Can you work these out from the drawing? Everything is in mm from the part's minimum corner. A direction names the side the tool comes from. Coordinates: 2 decimals unless noted, no trailing zeros. Write each loop counter-clockwise with the first axis right and the second up, starting at its lowest first coordinate (ties: lowest second). Pieces come first, ordered by that corner, then holes. Notation, with made-up numbers: (88, 85.25) -> (108, 85.25) arc R9 ccw to (108, 90.25) -> close; hole circle Ø3 at (-9.5, 88). An arc over 180 degrees is marked (long way). Use CSV: the item, a comma, the result in double quotes. Start each with the question number.
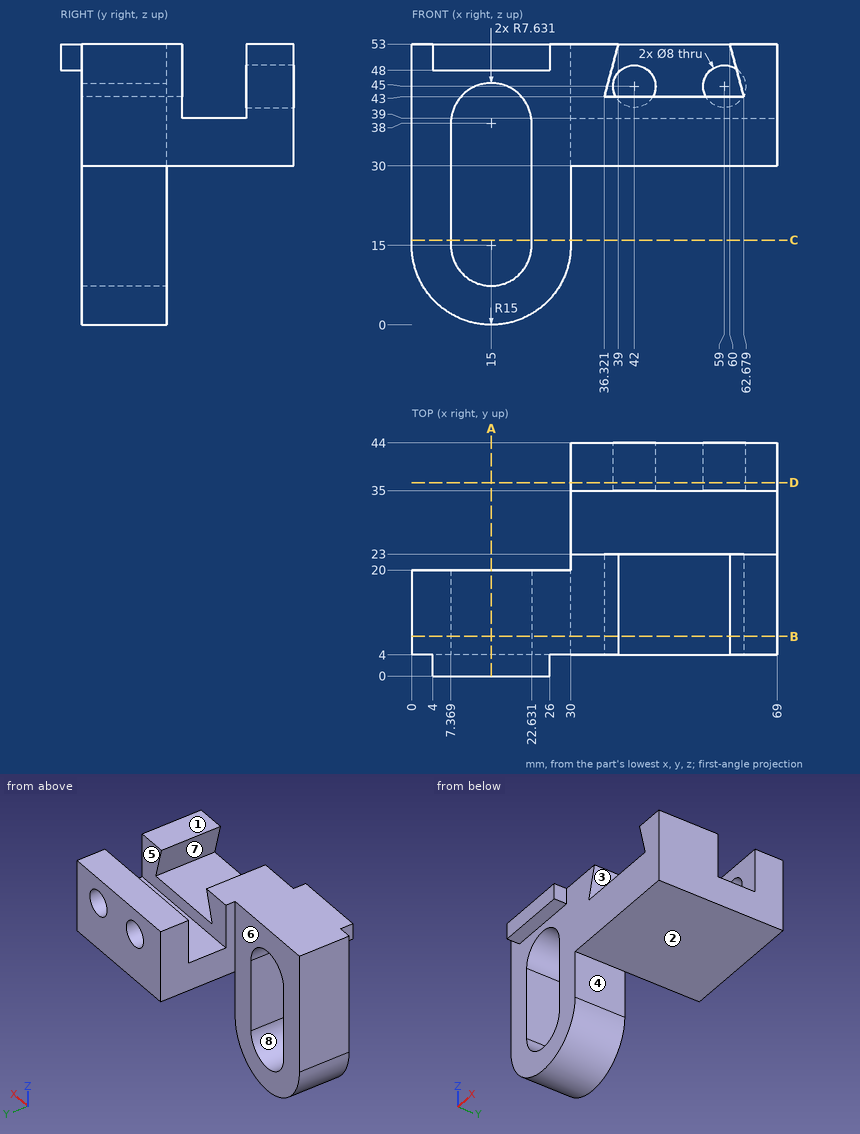
Item 1: I want a section at C-C on z = 16. Please give me the cut outline in (x, y).
Item 2: Thinking about a two-plate mould opening in Z: for the marked faces 1, 2 and 3, which applies, +Z half, -Z half, draft (parallel to the pull), parting line (faces both ways), or undercut?
Item 3: I'm going to push flat-ended pins straight in: pin 1 (10 mm diameter, centred on x = 56, y = 32, fed in from -Z); pin 2 (1.2 mm diameter, centred on y = 2, z = 51, fed in from -X); pin 3 (6.5 mm diameter, centred on x = 59, z = 45, fed in from +Y). Where does each tip first touch, or does it pass through?
Item 4: Which directions (+Z, -Z, +X, -X, +Y, -Y) give clear straight access to the entire face, cutting with the end or side of a thin tool? Please do the marked faces 4, 5, 6, 7 and 8.
Item 5: I want a section at A-A on x = 15. Please give me the cut outline in (y, z), then the cut area to 3 significant figures.
Item 6: I want a section at B-B on y = 7.5. Please give me the cut outline in (x, z), then the cut area to 3 significant figures.
Item 7: If I drill on line 1 along X through (y, z) = (38.5, 45); line 2 along X through (y, z) = (7.5, 35.5); line 3 along X through (y, z) = (7, 45) (1 decimal), over which ranges is the centre line in solid material (lowest first)?
Item 8: I want a section at D-D on y = 36.5. Please give me the cut outline in (x, z).
Geometry says:
1,outline,"(0, 4) -> (7.37, 4) -> (7.37, 20) -> (0, 20) -> close; (22.63, 4) -> (30, 4) -> (30, 20) -> (22.63, 20) -> close"
2,face 1,"+Z half"
2,face 2,"-Z half"
2,face 3,"undercut"
3,pin 1,"z = 30"
3,pin 2,"x = 4"
3,pin 3,"y = 23"
4,face 4,"-Z, +X, +Y, -Y"
4,face 5,"+Z, +X, -X"
4,face 6,"+Z, -Z, -X, +Y"
4,face 7,"-Y"
4,face 8,"+Y, -Y"
5,outline,"(0, 48) -> (4, 48) -> (4, 45.63) -> (20, 45.63) -> (20, 53) -> (0, 53) -> close; (4, 0) -> (20, 0) -> (20, 7.37) -> (4, 7.37) -> close"
5,area,"256 mm2"
6,outline,"(0, 15) arc R15 ccw to (30, 15) -> (30, 30) -> (69, 30) -> (69, 53) -> (60, 53) -> (62.68, 43) -> (36.32, 43) -> (39, 53) -> (0, 53) -> close; hole (7.37, 15) arc R7.63 ccw to (22.63, 15) -> (22.63, 38) arc R7.63 ccw to (7.37, 38) -> close"
6,area,"1,620 mm2"
7,line 1,"30 to 38, 46 to 55, 63 to 69"
7,line 2,"0 to 7.37, 22.63 to 69"
7,line 3,"0 to 12, 18 to 36.9, 62.1 to 69"
8,outline,"(30, 30) -> (69, 30) -> (69, 53) -> (30, 53) -> close; hole circle Ø8 at (42, 45); hole circle Ø8 at (59, 45)"
